For this review, take the finished solid that the model builds, in its own axes (mm). A direction names the side the tool comes from. Give positions to 0.01 mm unless a question says otherwise; leave off trailing zeros. Write each loop counter-clockwise with the first axis right and the second up, starting at its lowest first coordinate (ties: lowest second). Pieces come first, ordered by that corner, then holes.
1) Draft analysis for pull direction Y (two halves, no side actions). For faces 1 (the face through (0, 17, 28)), 2 (the face through (23.696, 9.492, 7.972)), 3 (the face through (-18.069, 12.831, -26.044)), state which applies: pulls with the +Y half, pulls with the -Y half, needs draft (parallel to the pull), parting line crosses it, or undercut.
2) Wall thickness on line 1 along Y through (x, z) = (-16.5, 18); line 2 along X through (y, z) = (11.5, 29.5); line 3 along X through (y, z) = (5.5, -11): over which ranges is each line inside the solid? List them lowest first.
3) For P1, Ø5, axis at x = 0.01, y = 11.5, coming from the -Z side; P2, Ø5, axis at x = 28, y = 9, coming from the -Z side; P3, Ø10, axis at y = 16.5, z = -16.5, coming from the -X side, all flat-tipped, find the tip position at first contact; note any pin that passes through.
4) We need section B-B on x = -8.5. Give the boundary of the cut face in (y, z), and give its area (3 significant figures).
5) Machinability: for faces 4 (the face through (-36.223, 9.86, 12.115)), 5 (the face through (5.39, 18.48, 29.04)), which of the approach directions +Z, -Z, +X, -X, +Y, -Y give a long, thin tool a straight path to every point of the face, cutting with its end or side? Answer none if there is none.
Autodesk Fusion 360 part; units mm, degrees
sketch "草图1" plane through (0, 0, 0) normal (0, 1, 0) x (1, 0, 0)
  circle A0 centre (0, 0) radius 15
  line L0 (18.1586, -25.0036) -> (29.3912, 9.5433)
  line L1 (29.3912, 9.5433) -> (0.0061, 30.9017)
  line L2 (0.0061, 30.9017) -> (-29.3874, 9.555)
  line L3 (-29.3874, 9.555) -> (-18.1685, -24.9964)
  line L4 (-18.1685, -24.9964) -> (18.1586, -25.0036)
  arc A1 (29.3912, 9.5433) -> (0.0061, 30.9017) centre (11.2288, 15.4486) ccw
  dimension "d1" = 30
  dimension "d2" = 25
extrude "拉伸1" add sketch "草图1" along normal blind 20 contours L1 A1 makes body 1
pattern_circular "C-阵列1" count 5 over 360 about axis through (0, 0, 0) along (0, 1, 0) of bodies 1 makes body 2 at (-14.2646, 13.3333, -34.3076) makes body 3 at (-31.7135, 13.3333, 19.3583) makes body 4 at (8.6108, 13.3333, 36.1433) makes body 5 at (19.0994, 6.6667, 24.9806)
extrude "拉伸2" add sketch "草图1" along normal blind 3 contours A0 | L0 L1 L2 L3 L4 bodies 1 2 3 4 5
cylinder "圆柱体基本要素1" add diameter 3 height 60 placed x (1, 0, 0) y (0, 1, 0) z (0, 0, 1) at (90, 0, 0) separate body makes body 6
move_body "对齐1" bodies 6 to x (-1, 0, -0.000199) y (0, -1, 0) z (-0.000199, 0, 1) at (90.007, 11.5, -34.9821)
move_body "移动1" bodies 6 to x (1, 0, 0) y (0, 1, 0) z (0, 0, 1) at (0, 0, 40)
pattern_circular "C-阵列2" count 5 over 360 about axis through (0, 0, 0) along (0, 1, 0) of bodies 6 makes body 7 at (42.3357, 11.6494, 15.3261) makes body 8 at (14.8431, 10.0116, -20.1175) makes body 9 at (-13.894, 10.3753, -20.8069) makes body 10 at (-23.5242, 12.76, 8.5023)
combine "合并1" operation cut target body 1 tool bodies 6 8 10 9 7
sketch "草图3" plane through (0, 0, 0) normal (0, 1, 0) x (1, 0, 0)
  line L0 (69.9416, -30.9016) -> (99.3712, -9.6047)
  line L1 (99.3712, -9.6047) -> (88.2108, 24.9656)
  line L2 (88.2108, 24.9656) -> (51.8837, 25.0343)
  line L3 (51.8837, 25.0343) -> (40.5927, -9.4936)
  line L4 (40.5927, -9.4936) -> (69.9416, -30.9016)
  point P0 (70, 0)
  dimension "d13" = 25
extrude "拉伸3" add sketch "草图3" along normal blind 3 separate body makes body 11
move_body "对齐2" bodies 11 to x (1, 0, 0) y (0, 1, 0) z (0, 0, 1) at (-69.9819, -3, -2.9337)
move_body "移动2" bodies 11 to x (1, 0, 0) y (0, 1, 0) z (0, 0, 1) at (0, 20, 0)
move_body "移动3" bodies 11 to x (1, 0, 0) y (0, 1, 0) z (0, 0, 1) at (0, 0, 5)
combine "合并2" operation cut target body 1 tool bodies 11
Results list:
1. face 1: pulls with the +Y half
1. face 2: needs draft
1. face 3: undercut
2. line 1: y = 0 to 3
2. line 2: x = -16.02 to -1.5, 1.5 to 16.01
2. line 3: x = -29.79 to -27.4, 27.39 to 29.8
3. P1: stops at z = -32.44
3. P2: stops at z = -28.14
3. P3: stops at x = -30.32
4. outline: (0, -34.36) - (20, -34.36) - (20, -24.72) - (3, -24.72) - (3, 25) - (17, 25) - (17, 26.8) - (20, 26.8) - (20, 36.2) - (0, 36.2) - close
4. area: 561 mm2
5. face 4: -X, +Y, -Y
5. face 5: +Y
